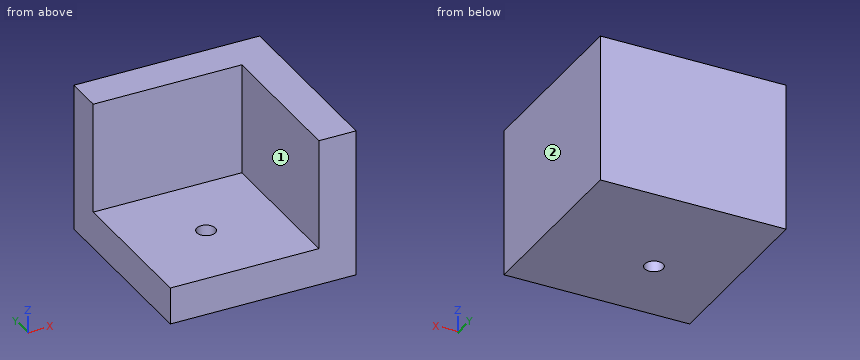
```python
from build123d import *

# Parameters (mm, degrees)
F0_W     = 31.75
F0_H     = 31.75
F1_DEPTH = 25.4
F2_W     = 25.4
F2_H     = 25.4
F3_DEPTH = 19.05
F5_D     = 3.175


with BuildPart() as f1:
    # F0 (on Top) → F1 (new body)
    with BuildSketch(Plane.XY):
        with Locations((15.875, 15.875)):
            Rectangle(F0_W, F0_H)
    extrude(amount=F1_DEPTH)

    # F2 (on face) → F3 (cut)
    with BuildSketch(Plane.XY.offset(25.4)):
        with Locations((12.7, 12.7)):
            Rectangle(F2_W, F2_H)
    extrude(amount=-F3_DEPTH, mode=Mode.SUBTRACT)

    # F5 (through all)
    with Locations(Plane.XY.offset(6.35)):
        with Locations((12.7, 12.7)):
            Hole(F5_D / 2)


solid = f1.part
```
The listing builds one solid part. Answer for the finished solid, in the listing's coordinates (mm). Face numbers are marked on the shaded views. A direction names the side the tool comes from. Round coordinates to 2 decimals unless told otherwise and drop trailing zeros. Loops run counter-clockwise (first coordinate to the right, second up) from the corner with the lowest first, then second, coordinate; pieces in that order, holes last.
Q1. Section A-A, the plane y = 12.7 is taken. Determine the outline of the cut face in (x, z).
Q2. Given pin 1 Ø9.5 at (y, z) = (7, 12) entering from -X; pin 2 Ø2 at (x, z) = (17, 10) entering from -Y; pin 3 Ø12.5 at (x, y) = (13.5, 11.5) entering from +Z, each flat-ended and moving along its own axis, determine where each tip first touches the part or whether it passes through.
Q3. Which of the six approach directions +Z, -Z, +X, -X, +Y, -Y give full straight-line access (tool end or side, diameter ignored) to the marked faces 1 and 2?
Q4. Find the intervals of material crossed by line 1 (Y direction, x = 12.7, z = 3.75); line 2 (X direction, y = 19, z = 7.5), in increasing order.
Q5. Section C-C, the plane z = 17 is taken. Determine the outline of the cut face in (x, y), then the cut area to 3 significant figures.
Q6. Section D-D, the plane x = 3 is taken. Determine the outline of the cut face in (y, z), then the cut area to 3 significant figures.
Completed:
1. outline: (0, 0) - (11.11, 0) - (11.11, 6.35) - (0, 6.35) - close; (14.29, 0) - (31.75, 0) - (31.75, 25.4) - (25.4, 25.4) - (25.4, 6.35) - (14.29, 6.35) - close
2. pin 1: stops at x = 25.4
2. pin 2: stops at y = 25.4
2. pin 3: stops at z = 6.35
3. face 1: +Z, -X, -Y
3. face 2: +Z, -Z, +X, +Y, -Y
4. line 1: y = 0 to 11.11, 14.29 to 31.75
4. line 2: x = 25.4 to 31.75
5. outline: (0, 25.4) - (25.4, 25.4) - (25.4, 0) - (31.75, 0) - (31.75, 31.75) - (0, 31.75) - close
5. area: 363 mm2
6. outline: (0, 0) - (31.75, 0) - (31.75, 25.4) - (25.4, 25.4) - (25.4, 6.35) - (0, 6.35) - close
6. area: 323 mm2
